from build123d import *

# Parameters (mm, degrees)
BOSS_EXTRUDE1_DEPTH     = 180
CUT_EXTRUDE1_DEPTH      = 183.66909974
CUT_EXTRUDE1_DEPTH_BACK = 183.66909974
SKETCH2_R               = 2.75


with BuildPart() as part:
    # Sketch1 → Boss-Extrude1 (new, symmetric)
    with BuildSketch(Plane(origin=(0, 0, 0), x_dir=(0, 0, -1), z_dir=(1, 0, 0))):
        Polygon((0, 22), (0, 0), (22, 0), (22, -3), (-3, -3), (-3, 22), align=None)
    extrude(amount=BOSS_EXTRUDE1_DEPTH, both=True)

    # Sketch2 → Cut-Extrude1 (cut, two sides: drawn at the far end of the back side and taken through both)
    with BuildSketch(Plane(origin=(0, 0, 0), x_dir=(1, 0, 0), z_dir=(0, 1, 0)).offset(-CUT_EXTRUDE1_DEPTH_BACK)):
        with Locations(Location((-160, 11, 0), (0, 0, 270))):
            Circle(SKETCH2_R)
        with Locations(Location((-120, 11, 0), (0, 0, 270))):
            Circle(SKETCH2_R)
        with Locations(Location((-80, 11, 0), (0, 0, 270))):
            Circle(SKETCH2_R)
        with Locations(Location((-40, 11, 0), (0, 0, 270))):
            Circle(SKETCH2_R)
        with Locations(Location((0, 11, 0), (0, 0, 270))):
            Circle(SKETCH2_R)
        with Locations(Location((40, 11, 0), (0, 0, 270))):
            Circle(SKETCH2_R)
        with Locations(Location((80, 11, 0), (0, 0, 270))):
            Circle(SKETCH2_R)
        with Locations(Location((120, 11, 0), (0, 0, 270))):
            Circle(SKETCH2_R)
        with Locations(Location((160, 11, 0), (0, 0, 270))):
            Circle(SKETCH2_R)
    extrude(amount=CUT_EXTRUDE1_DEPTH + CUT_EXTRUDE1_DEPTH_BACK, mode=Mode.SUBTRACT)


solid = part.part
Could you check a few things on this model? Use its own coordinates, in mm. A direction names the side the tool comes from. Give positions to 0.01 mm unless a question says otherwise; leave off trailing zeros. Order: outer loops, then holes, each group sorted by start corner. A loop starts at its lowest first (then second) coordinate and runs counter-clockwise, first axis right, second up. Notation, with made-up numbers: (7.25, -40) - (31.25, -40) arc R19 ccw to (31.25, -29) - close; hole circle Ø5 at (47, 3). An arc over 180 degrees is marked (long way). One line per item, written item: value. Start each with the question number.
1. Thinking about a two-plate mould opening in Z: for faces 1 (the face through (3, -3, -10)), 2 (the face through (3, 9, 3)), 3 (the face through (117.315, -1.521, -11.596)), 4 (the face through (-122.685, -1.521, -11.596)), which applies, +Z half, -Z half, draft (parallel to the pull), parting line (faces both ways), or undercut?
2. For P1, Ø3.5, axis at x = 120, z = -11, coming from the +Y side; P2, Ø7, axis at x = -80, z = -11, coming from the +Y side; P3, Ø6.5, axis at x = 40.5, y = 15.5, coming from the -Z side, each with a flat end and sliding along its axis, tell me the tip position at first contact or that it passes through.
3. Imagine slicing it at C-C on y = 15.25. List the corners of the cut face in (x, z) for me.
4. Imagine slicing it at B-B on z = -17.25. List the corners of the cut face in (x, y) for me.
5. For faces 5 (the face through (-162.44, -1.52, -9.73)), 6 (the face through (3, 11, 0)), which set-ups out of +Z, -Z, +X, -X, +Y, -Y let a thin tool reach every point of the face, with its end or its side?
6. Imagine slicing it at A-A on x = 143. List the corners of the cut face in (y, z) for me.
7. If I drill on probe 1 along Z at (x, y) = (-160, -1.2); probe 2 along Z at (x, y) = (-124, 1.75); probe 3 along Y at (x, z) = (163.5, -9.75), over which ranges is the centre line in solid material (lowest first)?
Values:
1. face 1: draft
1. face 2: +Z half
1. face 3: undercut
1. face 4: undercut
2. P1: through
2. P2: y = 0
2. P3: z = 0
3. outline: (-180, 0) - (180, 0) - (180, 3) - (-180, 3) - close
4. outline: (-180, -3) - (180, -3) - (180, 0) - (-180, 0) - close
5. face 5: +Y, -Y
5. face 6: -Z, +X, -X, +Y
6. outline: (-3, -22) - (0, -22) - (0, 0) - (22, 0) - (22, 3) - (-3, 3) - close
7. probe 1: -22 to -13.75, -8.25 to 3
7. probe 2: 0 to 3
7. probe 3: -3 to 0
